from build123d import *

# Parameters (mm, degrees)
SKETCH_2_R          = 40
EXTRUDE_1_DEPTH     = 5
SKETCH_1_R          = 36.75
SKETCH_1_R_2        = 29.25
SKETCH_1_R_3        = 24.75
SKETCH_1_R_4        = 23.25
CUT_EXTRUDE_1_DEPTH = 2


with BuildPart() as part:
    # 草图2 → 凸台-拉伸1 (new body)
    with BuildSketch(Plane.XY):
        with Locations((0, 0.759664545)):
            Circle(SKETCH_2_R)
    extrude(amount=EXTRUDE_1_DEPTH)

    # 草图1 → 切除-拉伸1 (cut)
    # profile 1 of 2: a face of its own
    with BuildSketch(Plane.XY):
        with Locations((0, 0.759664545)):
            Circle(SKETCH_1_R)
        Circle(SKETCH_1_R_2, mode=Mode.SUBTRACT)
    # profile 2 of 2: a face of its own
    with BuildSketch(Plane.XY):
        Circle(SKETCH_1_R_3)
        Circle(SKETCH_1_R_4, mode=Mode.SUBTRACT)
    extrude(amount=CUT_EXTRUDE_1_DEPTH, mode=Mode.SUBTRACT)


solid = part.part
Work out the finished part from the listing and answer in its coordinate system (mm). A direction names the side the tool comes from. Give positions to 0.01 mm unless a question says otherwise; leave off trailing zeros. Write each loop counter-clockwise with the first axis right and the second up, starting at its lowest first coordinate (ties: lowest second). Pieces come first, ordered by that corner, then holes. Notation, with made-up numbers: M 46.5,57 L 85.5,57 A13 cw 85.5,78 Z; hole C 85.25,5 d4. An arc over 180 degrees is marked long. Answer as CSV lines item,"result".
Q1. The mould has two halves that part along X. Classify faces 3 (the flat face through (18, -32, 0)), 4 (the flat face through (-11, 28, 2)), 5 (the cylindrical face through (38.153, 12.775, 2.465)): +X half, -X half, draft (parallel to the pull), parting line (faces both ways), or undercut.
A:
face 3,"draft"
face 4,"undercut"
face 5,"parting line"
Q2. Given P1, Ø1, axis at x = -23, z = 2, coming from the -Y side; P2, Ø1.5, axis at y = 16.5, z = 2, coming from the +X side; P3, Ø2, axis at y = 27, z = 1.5, coming from the +X side, each flat-ended and moving along its own axis, determine where each tip first touches the part or whether it passes through.
A:
P1,"stops at y = -32.31"
P2,"stops at x = 37.08"
P3,"stops at x = 31.03"
Q3. A tool of negligible diameter and unlimited length cuts with its end or side. For faces 1 (the cylindrical face through (-6.341, -28.554, 0.986)), 2 (the flat face through (-24, 7, 0)), from which of +Z, -Z, +X, -X, +Y, -Y can it reach the whole face along a straight path? Write none if from no direction.
A:
face 1,"-Z"
face 2,"-Z, +X, -X, +Y, -Y"
Q4. Find the intervals of material crossed by probe 1 along Y at (x, z) = (0, 1.55); probe 2 along X at (y, z) = (20, 0.6); probe 3 along Z at (x, y) = (7.5, 23.5), in increasing order. Write a range as [from, to].
A:
probe 1,"y = [-39.24, -35.99], [-29.25, -24.75], [-23.25, 23.25], [24.75, 29.25], [37.51, 40.76]"
probe 2,"x = [-35.07, -31.31], [-21.34, -14.58], [-11.86, 11.86], [14.58, 21.34], [31.31, 35.07]"
probe 3,"z = [2, 5]"
Q5. A cutting plane is placed at D-D on x = 31. Write down the section's boundary in (y, z), plus the area to 3 significant figures.
A:
outline,"M -24.52,0 L -18.98,0 L -18.98,2 L 20.5,2 L 20.5,0 L 26.04,0 L 26.04,5 L -24.52,5 Z"
area,"174 mm²"
Q6. A cutting plane is placed at A-A on x = 0. Write down the section's boundary in (y, z), plus the area to 3 significant figures.
A:
outline,"M -39.24,0 L -35.99,0 L -35.99,2 L -29.25,2 L -29.25,0 L -24.75,0 L -24.75,2 L -23.25,2 L -23.25,0 L 23.25,0 L 23.25,2 L 24.75,2 L 24.75,0 L 29.25,0 L 29.25,2 L 37.51,2 L 37.51,0 L 40.76,0 L 40.76,5 L -39.24,5 Z"
area,"364 mm²"
Q7. A cutting plane is placed at B-B on z = 1.25. Write down the section's boundary in (x, y).
A:
outline,"C 0,0.76 d80; C 0,0 d58.5; C 0,0 d46.5; hole C 0,0.76 d73.5; hole C 0,0 d49.5"
Q8. A cutting plane is placed at C-C on y = 17. Write down the section's boundary in (x, z), plus the area to 3 significant figures.
A:
outline,"M -36.55,0 L -32.97,0 L -32.97,2 L -23.8,2 L -23.8,0 L -17.99,0 L -17.99,2 L -15.86,2 L -15.86,0 L 15.86,0 L 15.86,2 L 17.99,2 L 17.99,0 L 23.8,0 L 23.8,2 L 32.97,2 L 32.97,0 L 36.55,0 L 36.55,5 L -36.55,5 Z"
area,"320 mm²"
